Could you check a few things on this model? Use its own coordinates, in mm. A direction names the side the tool comes from. Give positions to 0.01 mm unless a question says otherwise; leave off trailing zeros. Order: outer loops, then holes, each group sorted by start corner. A loop starts at its lowest first (then second) coordinate and runs counter-clockwise, first axis right, second up.
from build123d import *

# Parameters (mm, degrees)
BOSS_EXTRUDE1_DEPTH = 2
SKETCH3_R           = 1
CUT_EXTRUDE1_DEPTH  = 3
BOSS_EXTRUDE3_START = 3
SKETCH4_R           = 4.5
BOSS_EXTRUDE3_DEPTH = 3
SKETCH5_R           = 3
CUT_EXTRUDE2_DEPTH  = 1


with BuildPart() as part:
    # Sketch1 → Boss-Extrude1 (new body)
    with BuildSketch(Plane.XY):
        with BuildLine():
            Line((6.441226576, 5.332197615), (-12.558773424, 7.332197615))
            ThreePointArc((-12.558773424, 7.332197615), (-17.058773424, 2.832197615), (-12.558773424, -1.667802385))
            Line((-12.558773424, -1.667802385), (6.441226576, 0.332197615))
            ThreePointArc((6.441226576, 0.332197615), (8.941226576, 2.832197615), (6.441226576, 5.332197615))
        make_face()
    extrude(amount=BOSS_EXTRUDE1_DEPTH)

    # Sketch3 → Cut-Extrude1 (cut)
    with BuildSketch(Plane.XY.offset(2)):
        with Locations((6.441226576, 2.832197615)):
            Circle(SKETCH3_R)
    extrude(amount=-CUT_EXTRUDE1_DEPTH, mode=Mode.SUBTRACT)

    # Sketch4 → Boss-Extrude3 (add)
    with BuildSketch(Plane(origin=(0, 0, 0), x_dir=(-1, 0, 0), z_dir=(0, 0, -1)).offset(BOSS_EXTRUDE3_START)):
        with Locations((12.558773424, 2.832197615)):
            Circle(SKETCH4_R)
    extrude(amount=-BOSS_EXTRUDE3_DEPTH)

    # Sketch5 → Cut-Extrude2 (cut)
    with BuildSketch(Plane.XY.offset(2)):
        with Locations((-12.558773424, 2.832197615)):
            Circle(SKETCH5_R)
    extrude(amount=-CUT_EXTRUDE2_DEPTH, mode=Mode.SUBTRACT)


solid = part.part
Item 1: Imagine slicing it at B-B on z = 0.35. List the corners of the cut face in (x, y) for me.
Findings:
outline: (-12.56, -1.67) - (6.44, 0.33) arc R2.5 ccw to (6.44, 5.33) - (-12.56, 7.33) arc R4.5 ccw to start; hole circle Ø2 at (6.44, 2.83)
Item 2: Imagine slicing it at D-D on z = -1.45. List the corners of the cut face in (x, y) for me, then the cut area to 3 significant figures.
Findings:
outline: circle Ø9 at (-12.56, 2.83)
area: 63.6 mm2
Item 3: Please list where these lines run through material, in increasing order: line 1 along X through (y, z) = (3, 0.35); line 2 along Z through (x, y) = (-7, 0.5); line 3 along X through (y, z) = (0.75, 1.6).
Findings:
line 1: x = -17.06 to 5.46, 7.43 to 8.94
line 2: z = 0 to 2
line 3: x = -16.55 to -14.72, -10.4 to 7.82
Item 4: Imagine slicing it at A-A on x = -13.75. List the corners of the cut face in (y, z) for me, then the cut area to 3 significant figures.
Findings:
outline: (-1.51, -3) - (7.17, -3) - (7.17, 2) - (5.59, 2) - (5.59, 1) - (0.08, 1) - (0.08, 2) - (-1.51, 2) - close
area: 37.9 mm2
Item 5: Imagine slicing it at C-C on y = -1. List the corners of the cut face in (x, z) for me.
Findings:
outline: (-14.92, -3) - (-10.2, -3) - (-10.2, 0) - (-6.21, 0) - (-6.21, 2) - (-14.92, 2) - close
Item 6: For pin 1 (1.5 mm diameter, centred on y = 4, z = -1, fed in from -X); pin 2 (2.5 mm diameter, centred on x = -2.5, y = 4.5, fed in from -Z); pin 3 (2 mm diameter, centred on y = 6, z = 0.5, fed in from +X), each with a flat end and sliding along its axis, tell me the tip position at first contact or that it passes through.
Findings:
pin 1: stops at x = -17.04
pin 2: stops at z = 0
pin 3: stops at x = 7.69
Item 7: For faces 1 (the cylindrical face through (-16.735, 4.507, -0.535)), 2 (the cylindrical face through (6.903, 1.945, 1.014)), 3 (the cylindrical face through (-9.697, 3.733, 1.507)), which set-ups out of +Z, -Z, +X, -X, +Y, -Y let a thin tool reach every point of the face, with its end or its side?
Findings:
face 1: -Z
face 2: +Z, -Z
face 3: +Z
